Verification items for this drawing (mm, ordinates from the low corner). A direction names the side the tool comes from. Coordinates: 2 decimals unless noted, no trailing zeros. Order: outer loops, then holes, each group sorted by start corner. A loop starts at its lowest first (then second) coordinate and runs counter-clockwise, first axis right, second up. Notation, with made-up numbers: M -29.5,56.25 L -2.5,56.25 A22 ccw -2.5,66.25 Z; hole C 8.5,-15 d6. An arc over 180 degrees is marked long. Write item = value, one per line.
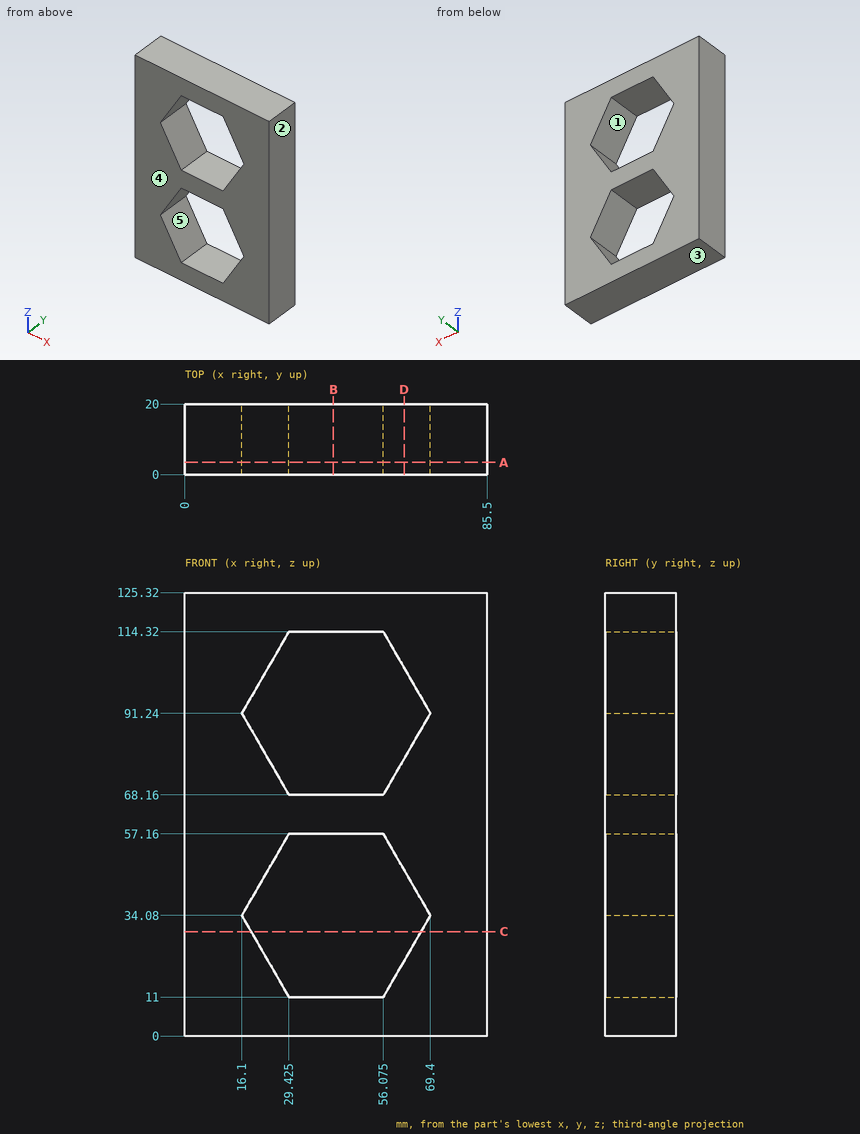
Item 1: Sectioned sample at C-C, the plane z = 29.5. Enter the section's corners in (x, y), then the cut area to 3 significant figures.
Report:
outline = M 0,0 L 18.74,0 L 18.74,20 L 0,20 Z; M 66.76,0 L 85.5,0 L 85.5,20 L 66.76,20 Z
area = 750 mm^2
Item 2: Sectioned sample at D-D, the plane x = 62. Enter the section's corners in (y, z), then the cut area to 3 significant figures.
Report:
outline = M 0,0 L 20,0 L 20,21.26 L 0,21.26 Z; M 0,46.9 L 20,46.9 L 20,78.42 L 0,78.42 Z; M 0,104.06 L 20,104.06 L 20,125.32 L 0,125.32 Z
area = 1,480 mm^2
Item 3: Tool access check on the marked faces 1 and 2. Record the directions out of +Z, -Z, +X, -X, +Y, -Y that give a thin tool (end or side, any length) a straight path to the whole face; none if there is none.
Report:
face_1 = +Y, -Y
face_2 = +Z, -Z, +X, +Y, -Y
Item 4: Scan lines: L1, parallel to Z at x = 32, y = 6.5; L2, parallel to Z at x = 57, y = 11.75 (1 decimal); L3, parallel to X at y = 12.25, z = 12. Record each from-to range of solid material in increasing order. Write a range as from..to.
Report:
L1 = 0..11, 57.16..68.16, 114.32..125.32
L2 = 0..12.6, 55.6..69.8, 112.7..125.3
L3 = 0..28.85, 56.65..85.5
Item 5: Release check for a two-part mould opening along Z. For the marked faces 3, 4 and 5 record: pulls with the +Z half, pulls with the -Z half, needs draft (parallel to the pull), parting line crosses it, or undercut.
Report:
face_3 = pulls with the -Z half
face_4 = needs draft
face_5 = undercut
Item 6: Sectioned sample at B-B, the plane x = 42. Enter the section's corners in (y, z), then the cut area to 3 significant figures.
Report:
outline = M 0,0 L 20,0 L 20,11 L 0,11 Z; M 0,57.16 L 20,57.16 L 20,68.16 L 0,68.16 Z; M 0,114.32 L 20,114.32 L 20,125.32 L 0,125.32 Z
area = 660 mm^2
Item 7: Sectioned sample at A-A, the plane y = 3.5. Enter the section's corners in (x, z) (1 decimal).
Report:
outline = M 0,0 L 85.5,0 L 85.5,125.3 L 0,125.3 Z; hole M 16.1,34.1 L 29.4,11 L 56.1,11 L 69.4,34.1 L 56.1,57.2 L 29.4,57.2 Z; hole M 16.1,91.2 L 29.4,68.2 L 56.1,68.2 L 69.4,91.2 L 56.1,114.3 L 29.4,114.3 Z
